Autodesk Inventor part; units mm, degrees
ref_plane "YZ Plane" through (0, 0, 0) normal (1, 0, 0) x (0, 1, 0)
ref_plane "XZ Plane" through (0, 0, 0) normal (0, 1, 0) x (-1, 0, 0)
ref_plane "XY Plane" through (0, 0, 0) normal (0, 0, 1) x (1, 0, 0)
sketch "Sketch1" plane through (0, 0, 0) normal (0, 0, 1) x (1, 0, 0)
  line L0 (-46, -175) -> (46, -175)
  line L1 (46, -175) -> (46, 175)
  line L2 (46, 175) -> (-46, 175)
  line L3 (-46, 175) -> (-46, -175)
  line L4 (-46, -175) -> (46, 175) construction
  line L5 (46, -175) -> (-46, 175) construction
  point P0 (0, 0)
  dimension "d154" = 92
  dimension "d155" = 350
extrude "Plate5" add sketch "Sketch1" along normal blind 2
sketch "Sketch7" plane through (-44, -175, 0) normal (-1, 0, 0) x (0, -1, 0)
  line L0 (-350, 0) -> (0, 0)
  line L1 (0, 0) -> (0, 94)
  line L2 (0, 94) -> (-350, 94)
  line L3 (-350, 94) -> (-350, 0)
edge flange "Flange3" height 94 angle 90 thickness 2 bend radius 2.75 thickness toward (-1, 0, 0) relief round relief width 2 relief depth 1 edges at (-46, 0, 2) wall of the first edge with corners at (-44, 175, 0) (-44, -175, 0) (-44, -175, 94) (-44, 175, 94)
bend "Bend3"
corner "Corner3"
sketch "Sketch8" plane through (0, 0, 2) normal (0, 0, 1) x (1, 0, 0)
  line L0 (46, 175) -> (46, -175)
  line L1 (-41.25, 175) -> (46, 175)
  line L2 (29, 170) -> (-27, 170)
  line L3 (-27, 170) -> (-27, 114)
  line L4 (-27, 114) -> (29, 114)
  line L5 (29, 114) -> (29, 170)
  line L6 (29, 170) -> (-27, 114) construction
  line L7 (-27, 170) -> (29, 114) construction
  point P0 (0, 0)
  point P1 (1, 142)
  point P2 (2.375, 175)
  dimension "d167" = 56
  dimension "d168" = 56
  dimension "d169" = 5
  dimension "d172" = 17
extrude "Cut1" cut sketch "Sketch8" against normal blind 2
properties part number "TZS 752 FDS 940 FLANGE 2" material "Stainless Steel"
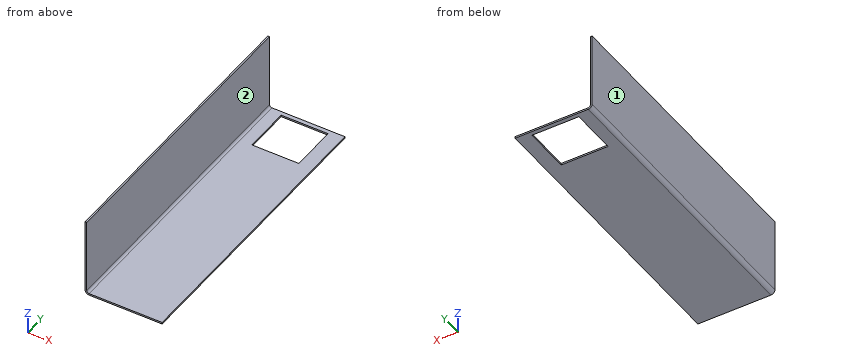
Design review of the part built by this model. Coordinates are the model's own, in mm. Face numbers are marked on the shaded views. A direction names the side the tool comes from. Give positions to 0.01 mm unless a question says otherwise; leave off trailing zeros. Write each loop counter-clockwise with the first axis right and the second up, starting at its lowest first coordinate (ties: lowest second). Pieces come first, ordered by that corner, then holes. Notation, with made-up numbers: (-9.75, -21) - (46.25, -21) arc R21 cw to (46.25, 12) - close; hole circle Ø4 at (72, 29). An arc over 180 degrees is marked (long way). Return JSON: item names as keys, results as strings. Group by question number.
(1) We need section A-A, the plane x = 22. Give the boundary of the cut face in (y, z), then the cut area to 3 significant figures.
(2) Machinability: for the marked faces 1 and 2, which of the approach directions +Z, -Z, +X, -X, +Y, -Y give a long, thin tool a straight path to every point of the face, cutting with its end or side? Answer none if there is none.
(3) To check wall thickness, follow probe 1 along Z at (x, y) = (16.5, -75); probe 2 along X at (y, z) = (35, 73); probe 3 along X at (y, z) = (95, 4). State the ranges of each line that lie inside material, in increasing order.
(4) Insertion check: pin 1 (1 mm diameter, centred on y = 147.5, z = 1, fed in from -X); pin 2 (5 mm diameter, centred on x = 3.5, y = 117.5, fed in from +Z); pin 3 (5 mm diameter, centred on x = 7, y = 115, fed in from +Z); pin 4 (3 mm diameter, centred on y = -47, z = 70.5, fed in from +X). Each pin has a flat end and moves straight along its axis. Give the tip position at first contact, or say it passes through.
(5) We need section B-B, the plane y = -95.5. Give the boundary of the cut face in (x, z), then the cut area to 3 significant figures.
(6) We need section D-D, the plane x = -37. Give the boundary of the cut face in (y, z), then the cut area to 3 significant figures.
(7) We need section C-C, the plane z = 29. Give the boundary of the cut face in (x, y).
Reported:
{
 "1": {"outline": "(-175, 0) - (114, 0) - (114, 2) - (-175, 2) - close; (170, 0) - (175, 0) - (175, 2) - (170, 2) - close", "area": "588 mm2"},
 "2": {"face 1": "+Z, -Z, -X, +Y, -Y", "face 2": "+Z, +X, +Y, -Y"},
 "3": {"probe 1": "z = 0 to 2", "probe 2": "x = -46 to -44", "probe 3": "x = -45.94 to -43.9"},
 "4": {"pin 1": "stops at x = -44.71", "pin 2": "passes through", "pin 3": "stops at z = 2", "pin 4": "stops at x = -44"},
 "5": {"outline": "(-46, 4.75) arc R4.75 ccw to (-41.25, 0) - (46, 0) - (46, 2) - (-41.25, 2) arc R2.75 cw to (-44, 4.75) - (-44, 94) - (-46, 94) - close", "area": "365 mm2"},
 "6": {"outline": "(-175, 0) - (175, 0) - (175, 2) - (-175, 2) - close", "area": "700 mm2"},
 "7": {"outline": "(-46, -175) - (-44, -175) - (-44, 175) - (-46, 175) - close"}
}
